Source: CAD feature listing. Evaluate the final solid. Frame: model axes, mm. Round coordinates to 2 decimals unless told otherwise and drop trailing zeros. Write each loop counter-clockwise with the first axis right and the second up, starting at its lowest first coordinate (ties: lowest second). Pieces come first, ordered by that corner, then holes.
from build123d import *

# Parameters (mm, degrees)
F1_DEPTH = 3.175


# Not quite as in the source:
# - ends of sketch curves that miss each other by under 0.0002 mm in the source are joined


with BuildPart() as f1:
    # F0 (on Front) → F1 (new body)
    with BuildSketch(Plane.XZ):
        with BuildLine():
            Line((256.8526232, -464.2309994), (318.5212324, -396.9739076))
            Line((318.5212324, -396.9739076), (235.5036438, -320.8543748))
            ThreePointArc((235.5036438, -320.8543748), (204.8703266123, -289.3256959733), (178.0726202767, -254.4783059859))
            Line((178.0726202767, -254.4783059859), (97.204276, -135.7211662))
            Line((97.204276, -135.7211662), (-84.3345278, 230.8220174))
            Line((-84.3345278, 230.8220174), (-195.8067712, 416.2626422))
            ThreePointArc((-195.8067712, 416.2626422), (-200.5384813212, 422.0145789545), (-206.7351977857, 426.1467211829))
            Line((-206.7351977857, 426.1467211829), (-282.2801314, 461.8011846))
            ThreePointArc((-282.2801314, 461.8011846), (-307.4924345817, 459.774434742), (-318.4536458896, 436.9792648454))
            Line((-318.4536458896, 436.9792648454), (-314.4572832, 382.307084))
            ThreePointArc((-314.4572832, 382.307084), (-313.9285810002, 379.4952234768), (-312.7838670978, 376.873066496))
            Line((-312.7838670978, 376.873066496), (63.4258828, -273.3887852))
            ThreePointArc((63.4258828, -273.3887852), (137.2742586369, -371.4240291313), (232.4799240247, -448.8861008552))
            Line((232.4799240247, -448.8861008552), (256.8526232, -464.2309994))
        make_face()
    extrude(amount=F1_DEPTH)


solid = f1.part
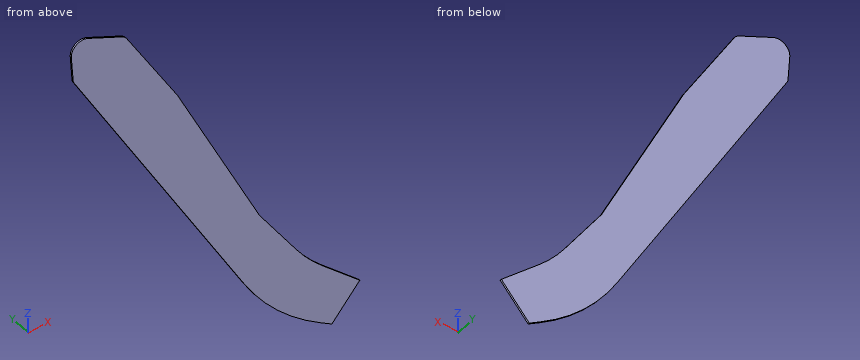
1) Section query A-A on y = -0.9. Return the cut outline in (x, z).
Taken from the geometry:
outline: (-318.45, 436.98) - (-314.46, 382.31) arc R12.7 ccw to (-312.78, 376.87) - (63.43, -273.39) arc R508 ccw to (232.48, -448.89) - (256.85, -464.23) - (318.52, -396.97) - (235.5, -320.85) arc R381 cw to (178.07, -254.48) - (97.2, -135.72) - (-84.33, 230.82) - (-195.81, 416.26) arc R25.4 ccw to (-206.74, 426.15) - (-282.28, 461.8) arc R25.4 ccw to start
2) Section query C-C on z = -239. Return the cut outline in (x, y) (3 decimals).
Taken from the geometry:
outline: (43.53, -3.175) - (167.533, -3.175) - (167.533, 0) - (43.53, 0) - close
3) Section query B-B on x = -170.5. Return the cut outline in (y, z) (3 decimals), then the cut area to 3 significant figures.
Taken from the geometry:
outline: (-3.175, 130.942) - (0, 130.942) - (0, 374.163) - (-3.175, 374.163) - close
area: 772 mm2
4) Material intervals for line 1 (Z direction, x = -55, y = -0.9); line 2 (Z direction, x = 148, y = -0.8); line 3 (X direction, y = -0.4, z = -218.5), sorted ascending.
Taken from the geometry:
line 1: z = -68.69 to 171.59
line 2: z = -382.23 to -210.32
line 3: x = 31.67 to 153.57
